Source: CAD feature listing. Evaluate the final solid. Frame: model axes, mm. Face numbers are marked on the shaded views. Round coordinates to 2 decimals unless told otherwise and drop trailing zeros. Loops run counter-clockwise (first coordinate to the right, second up) from the corner with the lowest first, then second, coordinate; pieces in that order, holes last. Notation, with made-up numbers: M -37.5,12 L -30.5,12 A29 ccw -30.5,34 Z; hole C 39.25,8 d1. An arc over 180 degrees is marked long. Write each question's results on one line, items separated by ' | '. Start each with the question number.
1. Ray query, line 1 (X direction, y = -53.5, z = 15); line 2 (X direction, y = -241.5, z = 5.75); line 3 (Y direction, x = -119, z = 4.25). Return the intervals inside material, ascending.
2. Section D-D on z = 16.5. Give the number of separate pieces and of enclosed holes in the cut face, and give its area (3 significant figures).
3. Section A-A on y = -133. Output: boundary loops of the cut face in (x, z).
4. Draft query along X for the marked faces 1 and 2. Return one class per face: released by +X, released by -X, zero draft, split by the parting line, or undercut.
5. Section B-B on x = -84. Output: boundary loops of the cut face in (y, z).
6. Contact query for flat-ended pins moving along their axis: pin 1 Ø13.5 at (y, z) = (-225.5, 8) entering from -X; pin 2 Ø5 at (y, z) = (-208.5, 11) entering from +X; pin 3 Ø5.5 at (y, z) = (-244.58, 5) entering from -X. Output: stop coordinate, or through.
7. Section C-C on y = -225. Output: boundary loops of the cut face in (x, z).
from build123d import *

# Parameters (mm, degrees)
BOSS_EXTRUDE1_DEPTH     = 25
BOSS_EXTRUDE2_DEPTH     = 2
BOSS_EXTRUDE3_DEPTH     = 27
SKETCH4_R               = 4.000000001
CUT_EXTRUDE1_DEPTH      = 290
CUT_EXTRUDE1_DEPTH_BACK = 10
BOSS_EXTRUDE4_DEPTH     = 27
SKETCH6_R               = 3.5
CUT_EXTRUDE2_DEPTH      = 108


with BuildPart() as part:
    # Sketch1 → Boss-Extrude1 (new body)
    with BuildSketch(Plane.XY):
        with BuildLine():
            Line((-199, 125.145211216), (-199, -165.423939983))
            ThreePointArc((-199, -165.423939983), (-181.870436917, -196.8510269), (-150.43197765, -213.959708975))
            Line((-150.43197765, -213.959708975), (150.431977646, -213.959708975))
            ThreePointArc((150.431977646, -213.959708975), (181.870436916, -196.8510269), (199, -165.423939981))
            Line((199, -165.423939981), (199, 125.145211216))
            ThreePointArc((199, 125.145211216), (182.477306779, 157.278075491), (150.333498342, 173.779467463))
            Line((150.333498342, 173.779467463), (-150.333498342, 173.779467463))
            ThreePointArc((-150.333498342, 173.779467463), (-182.477306779, 157.278075491), (-199, 125.145211216))
        make_face()
        with BuildLine():
            Line((-195, 124.810354463), (-195, -164.990595976))
            add(Edge.make_bspline(
                [(-195, -164.990595976), (-195, -209.959708976), (-150, -209.959708975)],
                knots=[3.141592654, 3.141592654, 3.141592654, 4.71238898, 4.71238898, 4.71238898], degree=2, weights=[1, 0.707106781, 1]))
            Line((-150, -209.959708975), (149.999999997, -209.959708975))
            add(Edge.make_bspline(
                [(149.999999997, -209.959708975), (195.000000002, -209.959708979), (195, -164.990595974)],
                knots=[4.71238898, 4.71238898, 4.71238898, 6.283185307, 6.283185307, 6.283185307], degree=2, weights=[1, 0.707106781, 1]))
            Line((195, -164.990595974), (195, 124.810354463))
            add(Edge.make_bspline(
                [(195, 124.810354463), (195, 169.779467463), (150, 169.779467463)],
                knots=[3.141592654, 3.141592654, 3.141592654, 4.71238898, 4.71238898, 4.71238898], degree=2, weights=[1, 0.707106781, 1]))
            Line((150, 169.779467463), (-150, 169.779467463))
            add(Edge.make_bspline(
                [(-150, 169.779467463), (-195, 169.779467463), (-195, 124.810354463)],
                knots=[1.570796327, 1.570796327, 1.570796327, 3.141592654, 3.141592654, 3.141592654], degree=2, weights=[1, 0.707106781, 1]))
        make_face(mode=Mode.SUBTRACT)
    extrude(amount=BOSS_EXTRUDE1_DEPTH)

    # Sketch2 → Boss-Extrude2 (add)
    with BuildSketch(Plane.XY.offset(25)):
        with BuildLine():
            Line((-199, 125.145211216), (-199, -165.423939983))
            ThreePointArc((-199, -165.423939983), (-181.870436917, -196.8510269), (-150.43197765, -213.959708975))
            Line((-150.43197765, -213.959708975), (150.431977646, -213.959708975))
            ThreePointArc((150.431977646, -213.959708975), (181.870436916, -196.8510269), (199, -165.423939981))
            Line((199, -165.423939981), (199, 125.145211216))
            ThreePointArc((199, 125.145211216), (182.477306779, 157.278075491), (150.333498342, 173.779467463))
            Line((150.333498342, 173.779467463), (-150.333498342, 173.779467463))
            ThreePointArc((-150.333498342, 173.779467463), (-182.477306779, 157.278075491), (-199, 125.145211216))
        make_face()
    extrude(amount=BOSS_EXTRUDE2_DEPTH)

    # Sketch3 → Boss-Extrude3 (add)
    with BuildSketch(Plane.XY.offset(27)):
        Polygon((-135, -204), (-135, -266.298841042), (-165, -266.298841042), (-180.688480604, -193.256655723), (-181.013326297, -190.888401224), (-177.05169199, -193.894319256), (-177.05169199, -195.902858929), (-162.575940018, -263.298841042), (-138, -263.298841042), (-138, -204), align=None)
    boss_extrude3 = extrude(amount=-BOSS_EXTRUDE3_DEPTH)

    # Mirror1: Boss-Extrude3 across plane
    add(boss_extrude3.mirror(Plane(origin=(0, 0, 0), x_dir=(0, 0, 1), z_dir=(1, 0, 0))))

    # Sketch4 → Cut-Extrude1 (cut, two sides)
    with BuildSketch(Plane(origin=(-135, 0, 0), x_dir=(0, 0, -1), z_dir=(1, 0, 0))) as cut_extrude1_sk:
        with Locations((-4.790160487, -266.968568277)):
            Circle(SKETCH4_R)
    extrude(amount=CUT_EXTRUDE1_DEPTH, mode=Mode.SUBTRACT)
    extrude(cut_extrude1_sk.sketch, amount=-CUT_EXTRUDE1_DEPTH_BACK, mode=Mode.SUBTRACT)

    # Sketch5 → Boss-Extrude4 (add)
    with BuildSketch(Plane.XY.offset(27)):
        Polygon((-46.130462584, -213.959708975), (-46.130462584, -250.580628677), (-42.5, -249.943543539), (-42.5, -213.959708975), align=None)
        Polygon((46.130462584, -250.580628677), (42.5, -249.943543539), (42.5, -213.959708975), (46.130462584, -213.959708975), align=None)
    extrude(amount=-BOSS_EXTRUDE4_DEPTH)

    # Sketch6 → Cut-Extrude2 (cut)
    with BuildSketch(Plane(origin=(46.130462584, 0, 0), x_dir=(0, 0, -1), z_dir=(1, 0, 0))):
        with Locations((-4.999999906, -244.580628739)):
            Circle(SKETCH6_R)
    extrude(amount=-CUT_EXTRUDE2_DEPTH, mode=Mode.SUBTRACT)


solid = part.part
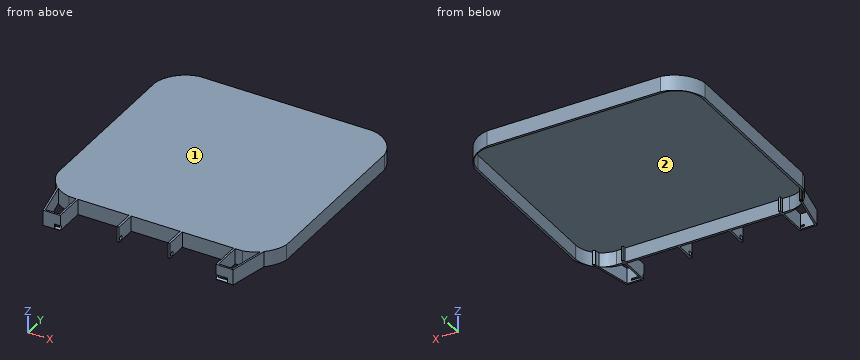
Taken from the geometry:
1) line 1: -199 to -195, 195 to 199 | line 2: -170.33 to -167.26, -138 to -135, 135 to 138, 167.26 to 170.33 | line 3: -213.96 to -209.96, 169.78 to 173.78
2) separate pieces: 1 | enclosed holes: 3 | area: 6,420 mm^2
3) outline: M -199,0 L -195,0 L -195,25 L 195,25 L 195,0 L 199,0 L 199,27 L -199,27 Z
4) face 1: zero draft | face 2: undercut
5) outline: M -213.96,0 L -209.96,0 L -209.96,25 L 169.78,25 L 169.78,0 L 173.78,0 L 173.78,27 L -213.96,27 Z
6) pin 1: x = -175.21 | pin 2: x = 177.95 | pin 3: x = -170.26
7) outline: M -173.87,0 L -170.8,0 L -170.8,27 L -173.87,27 Z; M -138,0 L -135,0 L -135,27 L -138,27 Z; M -46.13,0 L -42.5,0 L -42.5,27 L -46.13,27 Z; M 42.5,0 L 46.13,0 L 46.13,27 L 42.5,27 Z; M 135,0 L 138,0 L 138,27 L 135,27 Z; M 170.8,0 L 173.87,0 L 173.87,27 L 170.8,27 Z
